The listing builds one solid part. Answer for the finished solid, in the listing's coordinates (mm). Face numbers are marked on the shaded views. Coordinates: 2 decimals unless noted, no trailing zeros. Order: outer loops, then holes, each group sorted by start corner. A loop starts at its lowest first (then second) coordinate and runs counter-clockwise, first axis right, second up. Notation, with made-up numbers: (-27, 67) -> (25, 67) arc R35 cw to (25, 104) -> close; hole circle Ø3 at (-18, 59.25). An arc over 180 degrees is marked (long way). One line per question, with ' | ' between items.
from build123d import *

# Parameters (mm, degrees)
SKETCH1_W             = 19.05
SKETCH1_H             = 27.7495
BOSS_EXTRUDE1_DEPTH   = 1.5875
F_0_80_TAPPED_HOLE1_D = 1.19126
SKETCH4_W             = 3.175
SKETCH4_H             = 0.9398
SKETCH4_H_2           = 1.016
SKETCH4_H_3           = 1.050029844
BOSS_EXTRUDE2_DEPTH   = 0.3175
BOSS_EXTRUDE3_DEPTH   = 0.3175
LPATTERN1_COUNT       = 5
LPATTERN1_PITCH       = 5.5499
SKETCH8_R             = 1.27
BOSS_EXTRUDE4_DEPTH   = 1.27


with BuildPart() as part:
    # Sketch1 → Boss-Extrude1 (new body)
    with BuildSketch(Plane.XY):
        Rectangle(SKETCH1_W, SKETCH1_H)
    extrude(amount=BOSS_EXTRUDE1_DEPTH)

    # #0-80 Tapped Hole1 (through all)
    with Locations(Plane.XY.offset(1.5875)):
        with Locations((0, -11.0998), (0, -5.5499), (0, 0), (0, 5.5499), (0, 11.0998)):
            Hole(F_0_80_TAPPED_HOLE1_D / 2)

    # Sketch4 → Boss-Extrude2 (add)
    with BuildSketch(Plane.XY.offset(1.5875)):
        with Locations((4.7625, -4.3688)):
            Rectangle(SKETCH4_W, SKETCH4_H)
        with Locations((-4.7625, -9.8806)):
            Rectangle(SKETCH4_W, SKETCH4_H_2)
        with Locations((-4.7625, -6.858)):
            Rectangle(SKETCH4_W, SKETCH4_H_2)
        with Locations((4.7625, -1.3843)):
            Rectangle(SKETCH4_W, SKETCH4_H_2)
        with Locations((-4.7625, 1.2192)):
            Rectangle(SKETCH4_W, SKETCH4_H_2)
        with Locations((-4.7625, 4.2418)):
            Rectangle(SKETCH4_W, SKETCH4_H_2)
        with Locations((4.7625, 6.786114922)):
            Rectangle(SKETCH4_W, SKETCH4_H_3)
        with Locations((4.7625, 9.825729844)):
            Rectangle(SKETCH4_W, SKETCH4_H_2)
    extrude(amount=BOSS_EXTRUDE2_DEPTH)

    # Sketch6 → Boss-Extrude3 (add)
    with BuildSketch(Plane.XY.offset(1.5875)):
        Polygon((4.7625, -10.447923864), (-4.7625, -10.481668166), (-4.7625, -11.751668166), (4.7625, -11.751668166), align=None)
    boss_extrude3 = extrude(amount=BOSS_EXTRUDE3_DEPTH)

    # LPattern1: Boss-Extrude3 ×5
    with Locations(*[(0, i * LPATTERN1_PITCH, 0) for i in range(1, LPATTERN1_COUNT)]):
        add(boss_extrude3)

    # Sketch8 → Boss-Extrude4 (add)
    with BuildSketch(Plane.XY.offset(1.905)):
        Circle(SKETCH8_R)
        with Locations((0, 5.5499)):
            Circle(SKETCH8_R)
    extrude(amount=BOSS_EXTRUDE4_DEPTH)


solid = part.part
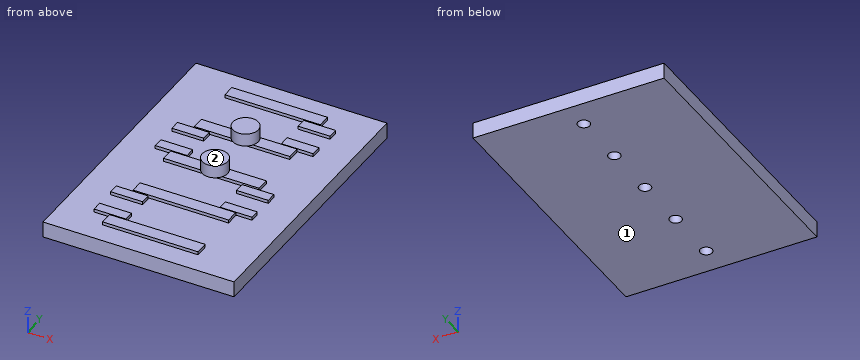
Item 1: Find the intervals of material crossed by L1, parallel to Y at x = 0, z = 1.2; L2, parallel to Y at x = -0.25, z = 0.35; L3, parallel to Z at x = -7.5, y = -9.5, in increasing order.
Computed values:
L1: y = -13.87 to -11.7, -10.5 to -6.15, -4.95 to -0.6, 0.6 to 4.95, 6.15 to 10.5, 11.7 to 13.87 | L2: y = -13.87 to -11.64, -10.56 to -6.09, -5.01 to -0.54, 0.54 to 5.01, 6.09 to 10.56, 11.64 to 13.87 | L3: z = 0 to 1.59
Item 2: Each of these flat-tipped pins is pushed along its axis until it touches: pin 1 Ø1 at (x, z) = (2.5, 3) entering from +Y; pin 2 Ø3 at (x, y) = (5.5, 2.5) entering from +Z; pin 3 Ø1 at (x, y) = (-1.5, -5.5) entering from +Z (3 decimals). Where does it stop, or does it pass through?
Computed values:
pin 1: passes through | pin 2: stops at z = 1.59 | pin 3: stops at z = 1.905
Item 3: Determine the mould class of the marked faces 1 and 2 for opening direction Z: pulls with the +Z half, pulls with the -Z half, needs draft (parallel to the pull), parting line crosses it, or undercut.
Computed values:
face 1: pulls with the -Z half | face 2: pulls with the +Z half
Item 4: Section C-C, the plane z = 2.3 is taken. Give the vertices of the cut face in (x, y), plus the area to 3 significant figures.
Computed values:
outline: circle Ø2.54 at (0, 0); circle Ø2.54 at (0, 5.55) | area: 10.1 mm^2
